from build123d import *

# Parameters (mm, degrees)
F0_R     = 33.7721508447
F1_DEPTH = 233.68
F2_DEPTH = 231.14
F3_DEPTH = 10.16


with BuildPart() as f1:
    # F0 (on Top) → F1 (new body)
    with BuildSketch(Plane.XY):
        Circle(F0_R)
    extrude(amount=-F1_DEPTH)

    # F2 (cut): a face of the model
    f2_faces = [f1.faces().sort_by_distance(p)[0] for p in [
        (0, 0, 0),
    ]]
    extrude(f2_faces, amount=-F2_DEPTH, mode=Mode.SUBTRACT)

    # F3 (add): a face of the model
    f3_faces = [f1.faces().sort_by_distance(p)[0] for p in [
        (0, 0, -233.68),
    ]]
    extrude(f3_faces, amount=F3_DEPTH)


solid = f1.part
Geometry: final body of the model. Coordinates: model frame, mm. Give positions to 0.01 mm unless a question says otherwise; leave off trailing zeros. Loops run counter-clockwise (first coordinate to the right, second up) from the corner with the lowest first, then second, coordinate; pieces in that order, holes last. Notation, with made-up numbers: (-17.75, 3) - (1.25, 3) arc R14 ccw to (1.25, 16) - close; hole circle Ø6 at (31, -20). An arc over 180 degrees is marked (long way). One line per question, with ' | ' between items. Start each with the question number.
(1) Section query B-B on x = 26.5. Return loops of the section in (y, z).
(2) Section query C-C on y = 14. Return loops of the section in (x, z).
(3) Ray query, line 1 (Y direction, x = 1, z = -239.75); line 2 (X direction, y = 23, z = -238); line 3 (Y direction, x = 26, z = -240.25). Return the intervals inside material, ascending. Write a range as from..to.
(4) Section query A-A on z = -234.75. Return loops of the section in (x, y), then the cut area to 3 significant figures.
(5) Contact query for flat-ended pins moving along their axis: pin 1 (6 mm diameter, centred on y = 16, z = -235.5, fed in from -X); pin 2 (1.5 mm diameter, centred on y = -24.5, z = -241, fed in from +X); pin 3 (2 mm diameter, centred on y = 20, z = -236, fed in from -X). Output: stop coordinate, or through.
The answers:
1) outline: (-20.94, -243.84) - (20.94, -243.84) - (20.94, -231.14) - (-20.94, -231.14) - close
2) outline: (-30.73, -243.84) - (30.73, -243.84) - (30.73, -231.14) - (-30.73, -231.14) - close
3) line 1: -33.76..33.76 | line 2: -24.73..24.73 | line 3: -21.55..21.55
4) outline: circle Ø67.54 at (0, 0) | area: 3,580 mm2
5) pin 1: x = -31.17 | pin 2: x = 24.01 | pin 3: x = -27.92
